The model under review builds one solid part; all positions refer to its coordinate system, in mm. A direction names the side the tool comes from. Round coordinates to 2 decimals unless told otherwise and drop trailing zeros. Answer as a JSON object with one key per item and string values. Group by question number.
1) Consider section A-A, the plane z = 0.25. Count the separate pieces of the cut face and the enclosed holes in it, then the cut area to 3 significant figures.
2) For faces 4 (the cylindrical face through (307.28, -239.464, 0.783)), 5 (the cylindrical face through (316.98, -160.89, 0.8)), list the 3-axis set-ups (+Z, -Z, +X, -X, +Y, -Y) from which the entire face can be reached by the end or side of a thin tool; tool diameter is ignored.
3) Insertion check: pin 1 Ø4.5 at (x, y) = (339.05, -185.81) entering from +Z. The pin has a flat end and moves straight along its axis. Give the tip position at first contact, or say it passes through.
4) To check wall thickness, follow line 1 (X direction, y = -75.5, z = 0.4); line 2 (X direction, y = -126.5, z = 0.2); line 3 (X direction, y = -147, z = 0.45). State the ranges of each line that lie inside material, in increasing order.
5) The part is to be moulded in two halves that separate along X. For faces 1 (the cylindrical face through (338.642, -196.293, 0.783)), 2 (the cylindrical face through (335.997, -196.056, 0.783)), 3 (the flat face through (280.77, -230.72, 0.78)), say which applies: +X half, -X half, draft (parallel to the pull), parting line (faces both ways), or undercut.
Autodesk Inventor part; units mm, degrees
ref_plane "YZ Plane" through (0, 0, 0) normal (1, 0, 0) x (0, 1, 0)
ref_plane "XZ Plane" through (0, 0, 0) normal (0, 1, 0) x (-1, 0, 0)
ref_plane "XY Plane" through (0, 0, 0) normal (0, 0, 1) x (1, 0, 0)
sketch "Sketch1" plane through (0, 0, 0) normal (0, 0, 1) x (1, 0, 0)
  circle A0 centre (241.6154, -140.1465) radius 2.4638
  arc A1 (259.0779, -181.0227) -> (259.0779, -99.2703) centre (241.6154, -140.1465) ccw
  line L0 (259.0779, -218.2466) -> (259.0779, -181.0227)
  arc A2 (312.3724, -235.9031) -> (359.2204, -154.9095) centre (11.2573, -7.6879) ccw
  arc A3 (359.2204, -154.9095) -> (360.17, -151.1328) centre (347.5241, -149.9609) ccw
  arc A4 (360.17, -151.1328) -> (262.8183, -22.9871) centre (241.6154, -140.1465) ccw
  arc A5 (301.8563, -242.8447) -> (312.3724, -235.9031) centre (241.6154, -140.1465) ccw
  arc A6 (262.8183, -22.9871) -> (259.0779, -26.1114) centre (262.2529, -26.1114) ccw
  line L1 (259.0779, -26.1114) -> (259.0779, -99.2703)
  line L2 (259.0779, -181.0227) -> (259.0779, -218.2466)
  circle A7 centre (268.2854, -38.5465) radius 2.1844
  circle A8 centre (268.2854, -216.3465) radius 2.1844
  arc A9 (308.9934, -232.4758) -> (354.8343, -153.0538) centre (11.2573, -7.6879) ccw
  arc A10 (354.8343, -153.0538) -> (355.4278, -150.6933) centre (347.5241, -149.9609) ccw
  arc A11 (355.4278, -150.6933) -> (263.8404, -28.0281) centre (241.6154, -140.1465) ccw
  circle A12 centre (263.8404, -28.0281) radius 2.413
  circle A13 centre (276.0241, -31.1486) radius 2.413
  circle A14 centre (287.7911, -35.5889) radius 2.413
  circle A15 centre (298.9991, -41.2951) radius 2.413
  circle A16 centre (309.5123, -48.1981) radius 2.413
  circle A17 centre (319.2034, -56.2144) radius 2.413
  circle A18 centre (327.9551, -65.247) radius 2.413
  circle A19 centre (335.6615, -75.1863) radius 2.413
  circle A20 centre (342.2292, -85.9122) radius 2.413
  circle A21 centre (347.5787, -97.2948) radius 2.413
  circle A22 centre (351.6452, -109.1961) radius 2.413
  circle A23 centre (354.3796, -121.4722) radius 2.413
  circle A24 centre (355.7487, -133.9744) radius 2.413
  circle A25 centre (355.7358, -146.5513) radius 2.413
  circle A26 centre (353.0365, -157.2317) radius 2.413
  circle A27 centre (348.7088, -166.7567) radius 2.413
  circle A28 centre (344.0523, -176.2817) radius 2.413
  circle A29 centre (339.0531, -185.8067) radius 2.413
  circle A30 centre (333.6952, -195.3317) radius 2.413
  circle A31 centre (327.9604, -204.8567) radius 2.413
  circle A32 centre (321.8278, -214.3817) radius 2.413
  circle A33 centre (315.2734, -223.9067) radius 2.413
  line L3 (301.8563, -242.8447) -> (259.0779, -218.2466)
  point P0 (259.0779, -22.3716)
  point P1 (295.3179, -246.41)
  dimension "d4" = 88.9
  dimension "d5" = 12.7
  dimension "d7" = 4.3688
  dimension "d8" = 4.7625
  dimension "d9" = 4.826
  dimension "d12" = 82
  dimension "d14" = 4.826
  dimension "d21" = 4.826
  dimension "d22" = 4.826
  dimension "d23" = 4.826
  dimension "d24" = 4.826
  dimension "d25" = 4.826
  dimension "d26" = 4.826
  dimension "d27" = 4.826
  dimension "d28" = 9.525
  dimension "d29" = 9.525
  dimension "d30" = 9.525
  dimension "d31" = 9.525
  dimension "d32" = 9.525
  dimension "d33" = 9.525
  dimension "d34" = 9.525
  dimension "d41" = 177.8
  dimension "d42" = 9.2075
extrude "Extrusion1" add sketch "Sketch1" along normal blind 1.5875 contours A1 L1 A6 A4 A3 A2 A5 L3 L0
sketch "Sketch4" plane through (0, 0, 1.5875) normal (0, 0, 1) x (1, 0, 0)
  point P0 (-212.5628, 245.6595)
sketch "Sketch6" plane through (0, 0, 1.5875) normal (0, 0, 1) x (1, 0, 0)
  circle A0 centre (263.8404, -28.0281) radius 2.413
  point P0 (0, 0)
extrude "Extrusion4" add sketch "Sketch6" against normal blind 1.5875
sketch "Sketch7" plane through (0, 0, 1.5875) normal (0, 0, 1) x (1, 0, 0)
  arc A0 (259.0779, -181.0227) -> (259.0779, -99.2703) centre (241.6154, -140.1465) ccw
  arc A1 (360.17, -151.1328) -> (262.8183, -22.9871) centre (241.6154, -140.1465) ccw
  arc A2 (359.2204, -154.9095) -> (360.17, -151.1328) centre (347.5241, -149.9609) ccw
  arc A3 (312.3724, -235.9031) -> (359.2204, -154.9095) centre (11.2573, -7.6879) ccw
  arc A4 (301.8563, -242.8447) -> (312.3724, -235.9031) centre (241.6154, -140.1465) ccw
  line L0 (259.0779, -218.2466) -> (301.8563, -242.8447)
  line L1 (259.0779, -181.0227) -> (259.0779, -218.2466)
  line L2 (259.0779, -26.1114) -> (259.0779, -99.2703)
  arc A5 (262.8183, -22.9871) -> (259.0779, -26.1114) centre (262.2529, -26.1114) ccw
  arc A6 (306.6939, -207.6622) -> (299.0406, -115.0702) centre (233.6747, -167.0854) ccw
  line L3 (304.5149, -208.2673) -> (286.208, -197.7406)
  arc A7 (285.7036, -195.4472) -> (296.3064, -116.6011) centre (215.7134, -145.8993) ccw
  arc A8 (331.0433, -153.7665) -> (275.984, -82.4202) centre (246.0316, -162.4533) ccw
  arc A9 (334.1816, -153.9043) -> (277.1253, -49.9392) centre (242.868, -136.3786) ccw
  arc A10 (331.0433, -153.7665) -> (334.1816, -153.9043) centre (332.6226, -153.6051) ccw
  arc A11 (299.0406, -115.0702) -> (296.3064, -116.6011) centre (297.7984, -116.0587) ccw
  line L4 (274.9529, -51.4151) -> (274.9529, -80.9334)
  arc A12 (277.1253, -49.9392) -> (274.9529, -51.4151) centre (276.5404, -51.4151) ccw
  arc A13 (274.9529, -80.9334) -> (275.984, -82.4202) centre (276.5404, -80.9334) ccw
  arc A14 (285.7036, -195.4472) -> (286.208, -197.7406) centre (286.9993, -196.3644) ccw
  arc A15 (304.5149, -208.2673) -> (306.6939, -207.6622) centre (305.3062, -206.8911) ccw
  point P0 (0, 0)
  point P1 (305.8979, -209.0626)
  point P2 (284.6802, -196.8621)
  point P3 (274.9529, -82.0418)
  point P4 (274.9529, -49.1096)
  dimension "d51" = 1.5875
  dimension "d52" = 1.5875
extrude "Extrusion5" cut sketch "Sketch7" against normal blind 1.5875 contours A15 L3 A14 A7 A11 A6 | A8 A13 L4 A12 A9 A10
properties part number "TopCurve"
Results list:
{
 "1": {"separate pieces": "1", "enclosed holes": "25", "area": "11,200 mm^2"},
 "2": {"face 4": "+Z, -Z, +X, -Y", "face 5": "+Z, -Z"},
 "3": {"pin 1": "through"},
 "4": {"line 1": "259.08 to 274.95, 313.15 to 333.27, 338.05 to 341.6", "line 2": "283.92 to 299.24, 306.69 to 323.55, 335.32 to 359.89", "line 3": "285.53 to 301.46, 314.76 to 330.08, 335.24 to 353.36, 358.11 to 360.48"},
 "5": {"face 1": "+X half", "face 2": "undercut", "face 3": "-X half"}
}
